```python
from build123d import *

# Parameters (mm, degrees)
F0_W     = 18.2
F0_H     = 2.6
F1_DEPTH = 11
F2_R     = 0.75
F3_DEPTH = 1.6
F4_R     = 0.75
F5_DEPTH = 1.6


with BuildPart() as f1:
    # F0 (on Top) → F1 (new body)
    with BuildSketch(Plane.XY):
        with Locations((9.1, 1.3)):
            Rectangle(F0_W, F0_H)
    extrude(amount=F1_DEPTH)

    # F2 (on face) → F3 (join)
    with BuildSketch(Plane.XY.offset(11)):
        with Locations((9.1, 1.3)):
            Circle(F2_R)
        with Locations((1.3, 1.3)):
            Circle(F2_R)
        with Locations((3.9, 1.3)):
            Circle(F2_R)
        with Locations((6.5, 1.3)):
            Circle(F2_R)
        with Locations((11.7, 1.3)):
            Circle(F2_R)
        with Locations((14.3, 1.3)):
            Circle(F2_R)
        with Locations((16.9, 1.3)):
            Circle(F2_R)
    extrude(amount=F3_DEPTH)

    # F4 (on face) → F5 (join)
    with BuildSketch(Plane(origin=(0, 0, 0), x_dir=(1, 0, 0), z_dir=(0, 0, -1))):
        with Locations((9.1, -1.3)):
            Circle(F4_R)
        with Locations((1.3, -1.3)):
            Circle(F4_R)
        with Locations((3.9, -1.3)):
            Circle(F4_R)
        with Locations((6.5, -1.3)):
            Circle(F4_R)
        with Locations((11.7, -1.3)):
            Circle(F4_R)
        with Locations((14.3, -1.3)):
            Circle(F4_R)
        with Locations((16.9, -1.3)):
            Circle(F4_R)
    extrude(amount=F5_DEPTH)


solid = f1.part
```
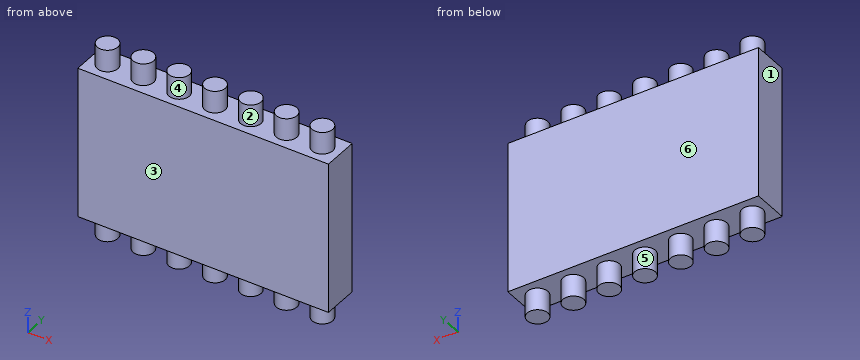
Here's how the part is built. I have some questions about the finished solid (model axes, mm). Face numbers are marked on the shaded views. A direction names the side the tool comes from. Coordinates: 2 decimals unless noted, no trailing zeros. Order: outer loops, then holes, each group sorted by start corner. A loop starts at its lowest first (then second) coordinate and runs counter-clockwise, first axis right, second up. Notation, with made-up numbers: M 74.25,-5 L 98.25,-5 A12 cw 98.25,2 Z; hole C -2,55.5 d5. An arc over 180 degrees is marked long. Answer as a JSON object with one key per item and string values. Group by question number.
(1) If we mould it in two halves opening along X, with no side actions, what happens to the marked faces 1, 2 and 3? For each: released by +X, released by -X, zero draft, split by the parting line, or undercut.
(2) For pin 1 (0.8 mm diameter, centred on x = 13, y = 1, fed in from -Z), with a flat end and sliding along its axis, tell me the tip position at first contact or that it passes through.
(3) Suppose I cut it at A-A, the plane x = 14.3. Please give me the cut outline in (y, z).
(4) I need wall thicknesses on probe 1 along Z at (x, y) = (9.75, 0.75); probe 2 along Y at (x, z) = (14.5, 11.75). Which ranges of each line are inside material? Lowest first, please.
(5) Which directions (+Z, -Z, +X, -X, +Y, -Y) give clear straight access to the entire face, cutting with the end or side of a thin tool? Please do the marked faces 4, 5 and 6.
(6) Suppose I cut it at B-B, the plane x = 1.5. Please give me the cut outline in (y, z), then the cut area to 3 significant figures.
Values found:
{
 "1": {"face 1": "released by -X", "face 2": "undercut", "face 3": "zero draft"},
 "2": {"pin 1": "stops at z = 0"},
 "3": {"outline": "M 0,0 L 0.55,0 L 0.55,-1.6 L 2.05,-1.6 L 2.05,0 L 2.6,0 L 2.6,11 L 2.05,11 L 2.05,12.6 L 0.55,12.6 L 0.55,11 L 0,11 Z"},
 "4": {"probe 1": "z = 0 to 11", "probe 2": "y = 0.58 to 2.02"},
 "5": {"face 4": "+Z", "face 5": "-Z", "face 6": "+Z, -Z, +X, -X, +Y"},
 "6": {"outline": "M 0,0 L 0.58,0 L 0.58,-1.6 L 2.02,-1.6 L 2.02,0 L 2.6,0 L 2.6,11 L 2.02,11 L 2.02,12.6 L 0.58,12.6 L 0.58,11 L 0,11 Z", "area": "33.2 mm^2"}
}
